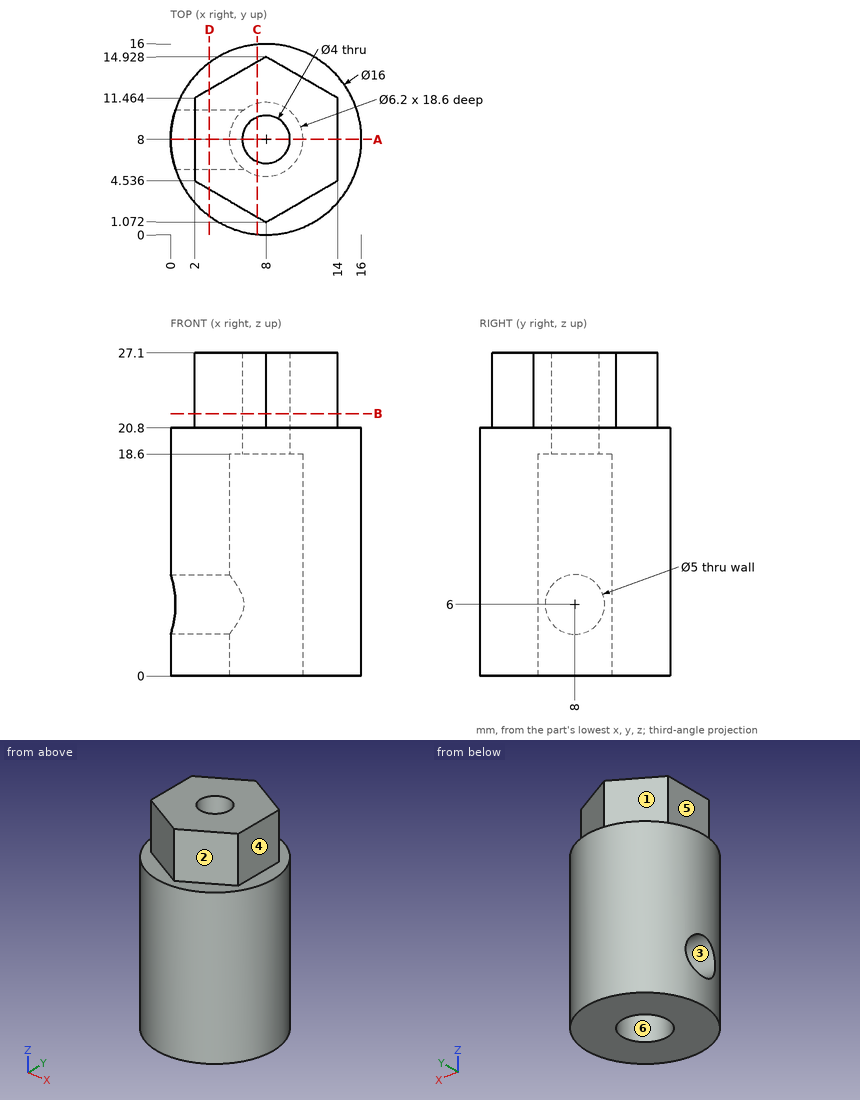
Geometry check sheet. Reference: drawing and pictorial views, mm from the part's lowest x, y, z. A direction names the side the tool comes from. Round coordinates to 2 decimals unless told otherwise and drop trailing zeros. Order: outer loops, then holes, each group sorted by start corner. A loop starts at its lowest first (then second) coordinate and runs counter-clockwise, first axis right, second up. Notation, with made-up numbers: (2, 67.25) -> (45, 67.25) arc R14 ccw to (45, 80.25) -> close; hole circle Ø3 at (19, 46). An arc over 180 degrees is marked (long way). One line per item, written item: value. Start each with the question number.
Q1. Cross-section at A-A (y = 8). Record the boundary of the cut face in (x, z), and give its area (3 significant figures).
Q2. Set-up check for the marked faces 4, 5 and 6: record each of +Z, -Z, +X, -X, +Y, -Y from which the full face is reachable in a straight line by a thin tool's end or side.
Q3. Thickness scan on line 1 (Y direction, x = 8, z = 5); line 2 (X direction, y = 4, z = 11.25); line 3 (Z direction, x = 3.5, y = 6). Record the ranges inside material, lowest first.
Q4. Gauge pin test, flat ends, axial feed: pin 1 Ø6 at (y, z) = (3, 9) entering from -X; pin 2 Ø4 at (y, z) = (8, 21.5) entering from +X; pin 3 Ø8 at (x, z) = (3, 24) entering from -Y; pin 4 Ø5 at (x, y) = (8, 8) entering from -Z. Record the tip position at first contact, or that the pin passes through.
Q5. Cross-section at C-C (x = 7.25). Record the boundary of the cut face in (y, z) (1 decimal), and give its area (3 significant figures).
Q6. Cross-section at B-B (z = 22). Record the boundary of the cut face in (x, y), and give its area (3 significant figures).
Q7. Mould release check, pull along Y, two halves, no side actions. Record for the marked faces 1, 2 and 3: pulls with the +Y half, pulls with the -Y half, needs draft (parallel to the pull), parting line crosses it, or undercut.
Q8. Cross-section at D-D (x = 3.25). Record the boundary of the cut face in (y, z), and give its area (3 significant figures).
Completed:
1. outline: (0, 0) -> (4.9, 0) -> (4.9, 3.5) -> (0, 3.5) -> close; (0, 8.5) -> (4.9, 8.5) -> (4.9, 18.6) -> (6, 18.6) -> (6, 27.1) -> (2, 27.1) -> (2, 20.8) -> (0, 20.8) -> close; (10, 18.6) -> (11.1, 18.6) -> (11.1, 0) -> (16, 0) -> (16, 20.8) -> (14, 20.8) -> (14, 27.1) -> (10, 27.1) -> close
1. area: 235 mm²
2. face 4: +Z, +X, +Y, -Y
2. face 5: +Z, -X, +Y, -Y
2. face 6: -Z
3. line 1: y = 0 to 4.9, 11.1 to 16
3. line 2: x = 1.07 to 14.93
3. line 3: z = 0 to 4.5, 7.5 to 27.1
4. pin 1: stops at x = 0.25
4. pin 2: stops at x = 16
4. pin 3: stops at y = 0.43
4. pin 4: stops at z = 18.6
5. outline: (0, 0) -> (5, 0) -> (5, 18.6) -> (6.1, 18.6) -> (6.1, 27.1) -> (1.5, 27.1) -> (1.5, 20.8) -> (0, 20.8) -> close; (9.9, 18.6) -> (11, 18.6) -> (11, 0) -> (16, 0) -> (16, 20.8) -> (14.5, 20.8) -> (14.5, 27.1) -> (9.9, 27.1) -> close
5. area: 270 mm²
6. outline: (2, 4.54) -> (8, 1.07) -> (14, 4.54) -> (14, 11.46) -> (8, 14.93) -> (2, 11.46) -> close; hole circle Ø4 at (8, 8)
6. area: 112 mm²
7. face 1: pulls with the +Y half
7. face 2: pulls with the -Y half
7. face 3: undercut
8. outline: (1.56, 0) -> (14.44, 0) -> (14.44, 20.8) -> (12.19, 20.8) -> (12.19, 27.1) -> (3.81, 27.1) -> (3.81, 20.8) -> (1.56, 20.8) -> close; hole circle Ø5 at (8, 6)
8. area: 301 mm²
